from build123d import *

# Parameters (mm, degrees)
SCHNITT_LINEAR_AUSTRAGEN1_REACH      = 179
SKIZZE3_R                            = 6
SCHNITT_LINEAR_AUSTRAGEN2_DEPTH      = 42.5
SCHNITT_LINEAR_AUSTRAGEN2_DEPTH_BACK = 42.5
SKIZZE4_R                            = 25
SCHNITT_LINEAR_AUSTRAGEN3_DEPTH      = 8
SKIZZE5_R                            = 15
SCHNITT_LINEAR_AUSTRAGEN4_DEPTH      = 20
KREISMUSTER1_COUNT                   = 4
SKIZZE9_R                            = 10
SCHNITT_LINEAR_AUSTRAGEN5_DEPTH      = 7.5
SCHNITT_LINEAR_AUSTRAGEN6_REACH      = 16.5
SKIZZE10_R                           = 7.5
SCHNITT_LINEAR_AUSTRAGEN7_REACH      = 27
SCHNITT_LINEAR_AUSTRAGEN8_REACH      = 27
SCHNITT_LINEAR_AUSTRAGEN8_END_RADIUS = 20
SKIZZE13_R                           = 4
SKIZZE14_R                           = 8
SCHNITT_LINEAR_AUSTRAGEN9_DEPTH      = 24
SKIZZE15_R                           = 8
SCHNITT_LINEAR_AUSTRAGEN10_DEPTH     = 24


with BuildPart() as part:
    # Skizze1 → Rotation1 (revolve)
    with BuildSketch(Plane(origin=(0, 0, 0), x_dir=(0, 0, -1), z_dir=(1, 0, 0)), mode=Mode.PRIVATE) as rotation1_sk:
        with BuildLine():
            Line((0, 0), (0, -38))
            Line((0, -38), (-2, -40))
            Line((-2, -40), (-50, -40))
            Line((-50, -40), (-50, -41.5))
            Line((-50, -41.5), (-65, -41.5))
            Line((-65, -41.5), (-89.84326674, -27.15673326))
            ThreePointArc((-89.84326674, -27.15673326), (-91.939425381, -22.096158641), (-97, -20))
            Line((-97, -20), (-175, -20))
            Line((-175, -20), (-177, -18))
            Line((-177, -18), (-177, -17))
            Line((-177, -17), (-176, -16))
            Line((-176, -16), (-86, -16))
            Line((-86, -16), (-76.386230096, 0))
            Line((-76.386230096, 0), (0, 0))
        make_face()
    revolve(rotation1_sk.sketch.rotate(Axis((0, 0, 212.688910887), (0, 0, -1)), 270), axis=Axis((0, 0, 212.688910887), (0, 0, -1)))  # turned: the seam where the file's is

    # Skizze2 → Schnitt-Linear austragen1 (cut, up to next)
    with BuildSketch(Plane(origin=(0, 0, 0), x_dir=(-1, 0, 0), z_dir=(0, 0, -1)), mode=Mode.PRIVATE) as schnitt_linear_austragen1_sk1:
        with BuildLine():
            Line((28.618176043, -25), (-28.618176043, -25))
            ThreePointArc((-28.618176043, -25), (0, -38), (28.618176043, -25))
        make_face()
    schnitt_linear_austragen1_tool1 = extrude(schnitt_linear_austragen1_sk1.sketch, amount=-SCHNITT_LINEAR_AUSTRAGEN1_REACH, mode=Mode.PRIVATE) & part.part
    add(schnitt_linear_austragen1_tool1.solids().sort_by_distance((0, -30.28468, 0))[0], mode=Mode.SUBTRACT)
    # Skizze2 → Schnitt-Linear austragen1 (cut, up to next)
    with BuildSketch(Plane(origin=(0, 0, 0), x_dir=(-1, 0, 0), z_dir=(0, 0, -1)), mode=Mode.PRIVATE) as schnitt_linear_austragen1_sk2:
        with BuildLine():
            ThreePointArc((28.618176043, 25), (0, 38), (-28.618176043, 25))
            Line((-28.618176043, 25), (28.618176043, 25))
        make_face()
    schnitt_linear_austragen1_tool2 = extrude(schnitt_linear_austragen1_sk2.sketch, amount=-SCHNITT_LINEAR_AUSTRAGEN1_REACH, mode=Mode.PRIVATE) & part.part
    add(schnitt_linear_austragen1_tool2.solids().sort_by_distance((0, 30.28468, 0))[0], mode=Mode.SUBTRACT)
    # Skizze2 → Schnitt-Linear austragen1 (cut, up to next)
    with BuildSketch(Plane(origin=(0, 0, 0), x_dir=(-1, 0, 0), z_dir=(0, 0, -1)), mode=Mode.PRIVATE) as schnitt_linear_austragen1_sk3:
        with BuildLine():
            ThreePointArc((33.749074061, 25), (0, 42), (-33.749074061, 25))
            Line((-33.749074061, 25), (-28.618176043, 25))
            ThreePointArc((-28.618176043, 25), (0, 38), (28.618176043, 25))
            Line((28.618176043, 25), (33.749074061, 25))
        make_face()
    schnitt_linear_austragen1_tool3 = extrude(schnitt_linear_austragen1_sk3.sketch, amount=-SCHNITT_LINEAR_AUSTRAGEN1_REACH, mode=Mode.PRIVATE) & part.part
    add(schnitt_linear_austragen1_tool3.solids().sort_by_distance((0, 38.69606, 0))[0], mode=Mode.SUBTRACT)
    # Skizze2 → Schnitt-Linear austragen1 (cut, up to next)
    with BuildSketch(Plane(origin=(0, 0, 0), x_dir=(-1, 0, 0), z_dir=(0, 0, -1)), mode=Mode.PRIVATE) as schnitt_linear_austragen1_sk4:
        with BuildLine():
            Line((-28.618176043, -25), (-33.749074061, -25))
            ThreePointArc((-33.749074061, -25), (0, -42), (33.749074061, -25))
            Line((33.749074061, -25), (28.618176043, -25))
            ThreePointArc((28.618176043, -25), (0, -38), (-28.618176043, -25))
        make_face()
    schnitt_linear_austragen1_tool4 = extrude(schnitt_linear_austragen1_sk4.sketch, amount=-SCHNITT_LINEAR_AUSTRAGEN1_REACH, mode=Mode.PRIVATE) & part.part
    add(schnitt_linear_austragen1_tool4.solids().sort_by_distance((31.183625, -25.69606, 0))[0], mode=Mode.SUBTRACT)

    # Skizze3 → Schnitt-Linear austragen2 (cut, two sides)
    with BuildSketch(Plane(origin=(0, 0, 0), x_dir=(0, 0, -1), z_dir=(1, 0, 0))) as schnitt_linear_austragen2_sk:
        with Locations((-32, 0)):
            Circle(SKIZZE3_R)
    extrude(amount=SCHNITT_LINEAR_AUSTRAGEN2_DEPTH, mode=Mode.SUBTRACT)
    extrude(schnitt_linear_austragen2_sk.sketch, amount=-SCHNITT_LINEAR_AUSTRAGEN2_DEPTH_BACK, mode=Mode.SUBTRACT)

    # Skizze4 → Schnitt-Linear austragen3 (cut)
    with BuildSketch(Plane(origin=(0, 25, 0), x_dir=(1, 0, 0), z_dir=(0, 1, 0))):
        with Locations(Location((0, -32, 0), (0, 0, 270))):  # turned: the seam where the file's is
            Circle(SKIZZE4_R)
    extrude(amount=-SCHNITT_LINEAR_AUSTRAGEN3_DEPTH, mode=Mode.SUBTRACT)

    # Skizze5 → Schnitt-Linear austragen4 (cut)
    with BuildSketch(Plane(origin=(0, 17, 0), x_dir=(1, 0, 0), z_dir=(0, 1, 0))):
        with Locations(Location((0, -32, 0), (0, 0, 270))):  # turned: the seam where the file's is
            Circle(SKIZZE5_R)
    extrude(amount=-SCHNITT_LINEAR_AUSTRAGEN4_DEPTH, mode=Mode.SUBTRACT)

    # Skizze7 → M4 Gewindebohrung1 (revolve, cut)
    with BuildSketch(Plane(origin=(-14.142135624, 17, 17.857864376), x_dir=(0, 0, 1), z_dir=(1, 0, 0))):
        Polygon((0, 0), (0, 12.491420021), (1.65, 11.5), (1.65, 0), align=None)
    m4_gewindebohrung1 = revolve(axis=Axis((-14.142135624, 23.35, 17.857864376), (0, -1, 0)), mode=Mode.SUBTRACT)

    # Kreismuster1: M4 Gewindebohrung1 ×4 about axis
    kreismuster1_axis = Axis((0, 0, 32), (0, 1, 0))
    for i in range(1, KREISMUSTER1_COUNT):
        add(m4_gewindebohrung1.rotate(kreismuster1_axis, i * 360 / KREISMUSTER1_COUNT), mode=Mode.SUBTRACT)

    # Skizze9 → Schnitt-Linear austragen5 (cut)
    with BuildSketch(Plane(origin=(0, -3, 0), x_dir=(1, 0, 0), z_dir=(0, 1, 0))):
        with Locations(Location((0, -32, 0), (0, 0, 270))):  # turned: the seam where the file's is
            Circle(SKIZZE9_R)
    extrude(amount=-SCHNITT_LINEAR_AUSTRAGEN5_DEPTH, mode=Mode.SUBTRACT)

    # Skizze10 → Schnitt-Linear austragen6 (cut, up to next)
    with BuildSketch(Plane(origin=(0, -10.5, 0), x_dir=(1, 0, 0), z_dir=(0, 1, 0)), mode=Mode.PRIVATE) as schnitt_linear_austragen6_sk1:
        with Locations(Location((0, -32, 0), (0, 0, 270))):  # turned: the seam where the file's is
            Circle(SKIZZE10_R)
    schnitt_linear_austragen6_tool1 = extrude(schnitt_linear_austragen6_sk1.sketch, amount=-SCHNITT_LINEAR_AUSTRAGEN6_REACH, mode=Mode.PRIVATE) & part.part
    add(schnitt_linear_austragen6_tool1.solids().sort_by_distance((0, -10.5, 32))[0], mode=Mode.SUBTRACT)

    # Skizze12 → Schnitt-Linear austragen7 (cut, up to next)
    with BuildSketch(Plane(origin=(0, 0, 0), x_dir=(1, 0, 0), z_dir=(0, 1, 0)), mode=Mode.PRIVATE) as schnitt_linear_austragen7_sk1:
        with BuildLine():
            Line((-4, -155), (-4, -177))
            Line((-4, -177), (4, -177))
            Line((4, -177), (4, -155))
            ThreePointArc((4, -155), (0, -151), (-4, -155))
        make_face()
    schnitt_linear_austragen7_tool1 = extrude(schnitt_linear_austragen7_sk1.sketch, amount=-SCHNITT_LINEAR_AUSTRAGEN7_REACH, mode=Mode.PRIVATE) & part.part
    add(schnitt_linear_austragen7_tool1.solids().sort_by_distance((0, 0, 164.413352))[0], mode=Mode.SUBTRACT)

    # Schnitt-Linear austragen8: up to this cylinder (the profile starts inside it)
    schnitt_linear_austragen8_end = Plane(origin=(0, 0, 137), z_dir=(0, 0, 1)) * Cylinder(SCHNITT_LINEAR_AUSTRAGEN8_END_RADIUS, 95, mode=Mode.PRIVATE)
    # Skizze13 → Schnitt-Linear austragen8 (cut, up to the surface)
    with BuildSketch(Plane(origin=(0, 0, 0), x_dir=(1, 0, 0), z_dir=(0, 1, 0)), mode=Mode.PRIVATE) as schnitt_linear_austragen8_sk1:
        with Locations(Location((0, -137, 0), (0, 0, 90))):  # turned: the seam where the file's is
            Circle(SKIZZE13_R)
    schnitt_linear_austragen8_tool1 = extrude(schnitt_linear_austragen8_sk1.sketch, amount=SCHNITT_LINEAR_AUSTRAGEN8_REACH, mode=Mode.PRIVATE) & schnitt_linear_austragen8_end
    add(schnitt_linear_austragen8_tool1.solids().sort_by_distance((0, 0, 137))[0], mode=Mode.SUBTRACT)

    # Skizze14 → Schnitt-Linear austragen9 (cut)
    with BuildSketch(Plane(origin=(40, 0, 2), x_dir=(0, 0, -1), z_dir=(1, 0, 0))):
        with Locations((-30, 0)):
            Circle(SKIZZE14_R)
    extrude(amount=-SCHNITT_LINEAR_AUSTRAGEN9_DEPTH, mode=Mode.SUBTRACT)

    # Skizze15 → Schnitt-Linear austragen10 (cut)
    with BuildSketch(Plane(origin=(-40, 0, 2), x_dir=(0, 0, 1), z_dir=(-1, 0, 0))):
        with Locations(Location((30, 0, 0), (0, 0, 180))):  # turned: the seam where the file's is
            Circle(SKIZZE15_R)
    extrude(amount=-SCHNITT_LINEAR_AUSTRAGEN10_DEPTH, mode=Mode.SUBTRACT)


solid = part.part
Can you work these out from the model? Positions are in its coordinate system, mm. A direction names the side the tool comes from. Coordinates: 2 decimals unless noted, no trailing zeros. Write each loop counter-clockwise with the first axis right and the second up, starting at its lowest first coordinate (ties: lowest second). Pieces come first, ordered by that corner, then holes. Notation, with made-up numbers: (-0.75, -27.75) -> (24.25, -27.75) arc R14 ccw to (24.25, -7.75) -> close; hole circle Ø7 at (32.5, 18.5). An arc over 180 degrees is marked (long way). Write each question's results on one line, items separated by ' | '. Start each with the question number.
Item 1: Please list where these lines run through material, in increasing order: probe 1 along Y at (x, z) = (-12, 115.5); probe 2 along Y at (x, z) = (14.5, 23); probe 3 along Z at (x, y) = (22.5, 14.5).
Item 2: If we section it at B-B, the plane z = 110: Write out the boundary of the cut face in (x, y).
Item 3: If we section it at C-C, the plane z = 53.5: Write out the boundary of the cut face in (x, y), and give its area (3 significant figures).
Item 4: On a 3-axis mill with a long thin cutter (end or side, diameter ignored), from which of +Z, -Z, +X, -X, +Y, -Y can I reach the whole of each face in a straight line? I mean faces 5 (the flat face through (0, -3, 43)), 6 (the cylindrical face through (40, 0, 21)), 7 (the flat face through (-4, -18, 166)). Say none if no direction works.
Item 5: Thinking about a two-plate mould opening in X: for faces 1 (the cylindrical face through (-40, 0, 21)), 2 (the conical face through (38.123, 0.383, 0.125)), 3 (the cylindrical face through (15.79, 11.33, 17.79)), 4 (the conical face through (-0.754, 18.304, 176.681)), which applies, released by +X, released by -X, zero draft, split by the parting line, or undercut?
Item 6: If we section it at A-A, the plane z = 32.5: Count the separate pieces of the cut face and the enclosed holes in it, and give its area (3 significant figures).
Item 7: If we section it at D-D, the plane z = 80.5: Write out the boundary of the cut face in (x, y).
Item 8: I'm going to push flat-ended pins straight in: P1, Ø5, axis at x = -0.5, z = 23, coming from the +Y side; P2, Ø8, axis at y = 1, z = 30, coming from the +X side; P3, Ø7, axis at y = 0, z = 32, coming from the +X side; P4, Ø12, axis at x = -8.5, z = 145, coming from the -Y side. Where does each tip first touch, or does it pass through?
Answer block:
1) probe 1: -16 to -10.58, 10.58 to 16 | probe 2: -25 to 17 | probe 3: 0 to 89.85
2) outline: circle Ø40 at (0, 0); hole circle Ø32 at (0, 0)
3) outline: (-33.12, -25) -> (33.12, -25) arc R41.5 ccw to (33.12, 25) -> (12.76, 25) -> (12.76, 17) -> (-12.76, 17) -> (-12.76, 25) -> (-33.12, 25) arc R41.5 ccw to start | area: 3,680 mm²
4) face 5: +Y | face 6: -Z, +X | face 7: +Z, -Y
5) face 1: released by -X | face 2: released by +X | face 3: undercut | face 4: split by the parting line
6) separate pieces: 4 | enclosed holes: 0 | area: 1,540 mm²
7) outline: (-20.85, -25) -> (20.85, -25) arc R32.55 ccw to (20.85, 25) -> (-20.85, 25) arc R32.55 ccw to start; hole circle Ø13.69 at (0, 0)
8) P1: y = -3 | P2: x = 16 | P3: through | P4: y = -19.84
